Could you check a few things on this model? Use its own coordinates, in mm. Face numbers are marked on the shaded views. A direction names the side the tool comes from. Round coordinates to 2 decimals unless told otherwise and drop trailing zeros. Loops run counter-clockwise (first coordinate to the right, second up) from the corner with the lowest first, then second, coordinate; pieces in that order, holes last. Notation, with made-up numbers: M -7.5,67.25 L -1.5,67.25 A8 cw -1.5,78.25 Z; hole C 20,25 d8. An arc over 180 degrees is marked long. Answer in a Markdown table with one row per item.
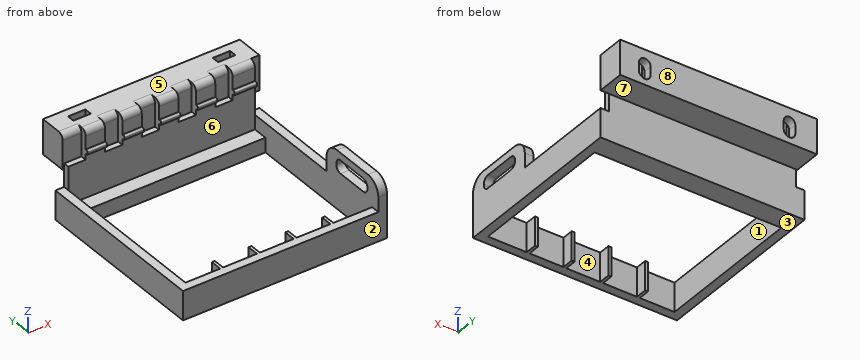
```python
from build123d import *

# Parameters (mm, degrees)
F0_W      = 70.5
F0_H      = 61.57
F0_W_2    = 1
F0_H_2    = 4
F1_DEPTH  = 10
F0_W_3    = 64.5
F0_H_3    = 5.07
F2_DEPTH  = 5
F3_W      = 64.5
F3_H      = 2
F4_DEPTH  = 18
F5_W      = 1
F5_H      = 1.5
F6_DEPTH  = 64.5
F7_R      = 0.5
F8_W      = 6
F8_H      = 9.142870052
F9_DEPTH  = 10
F10_W     = 9.5
F10_H     = 12
F11_DEPTH = 68
F13_DEPTH = 4
F14_W     = 6
F14_H     = 2.6
F15_DEPTH = 11
F17_DEPTH = 10
F18_W     = 15
F18_H     = 4.5
F19_DEPTH = 25
F20_R     = 5
F21_R     = 1.99999


# Not quite as in the source:
# - a fillet or chamfer is up to 0.001 mm smaller than in the source, because OpenCascade refuses the exact size


with BuildPart() as f1:
    # F0 (on Top) → F1 (new body)
    with BuildSketch(Plane.XY):
        with Locations((20.3630310733, 4.7424566842)):
            Rectangle(F0_W, F0_H)
        Polygon((-11.8869689267, 28.4574566842), (-11.8869689267, 33.5274566842), (52.6130310733, 33.5274566842), (52.6130310733, 28.4574566842), (52.6130310733, -23.0425433158), (39.2130310733, -23.0425433158), (38.2130310733, -23.0425433158), (26.5130310733, -23.0425433158), (25.5130310733, -23.0425433158), (13.8130310733, -23.0425433158), (12.8130310733, -23.0425433158), (1.1130310733, -23.0425433158), (0.1130310733, -23.0425433158), (-11.8869689267, -23.0425433158), align=None, mode=Mode.SUBTRACT)
        with Locations((0.6130310733, -21.0425433158)):
            Rectangle(F0_W_2, F0_H_2)
        with Locations((13.3130310733, -21.0425433158)):
            Rectangle(F0_W_2, F0_H_2)
        with Locations((26.0130310733, -21.0425433158)):
            Rectangle(F0_W_2, F0_H_2)
        with Locations((38.7130310733, -21.0425433158)):
            Rectangle(F0_W_2, F0_H_2)
    extrude(amount=F1_DEPTH)

    # F0 (on Top) → F2 (join)
    with BuildSketch(Plane.XY):
        with Locations((20.3630310733, 30.9924566842)):
            Rectangle(F0_W_3, F0_H_3)
    extrude(amount=F2_DEPTH)

    # F3 (on face) → F4 (join)
    with BuildSketch(Plane.XY.offset(10)):
        with Locations((20.3630310733, 34.5274566842)):
            Rectangle(F3_W, F3_H)
    extrude(amount=F4_DEPTH)

    # F5 (on face) → F6 (join)
    with BuildSketch(Plane.YZ.offset(52.6130310733)):
        with Locations((33.0274566842, 20.75)):
            Rectangle(F5_W, F5_H)
    extrude(amount=-F6_DEPTH)

    # F7
    f7_edges = [f1.edges().sort_by_distance(p)[0] for p in [
        (20.363031, 32.527457, 21.5),
        (20.363031, 32.527457, 20),
    ]]
    fillet(f7_edges, radius=F7_R)

    # F8 (on face) → F9 (cut)
    with BuildSketch(Plane.XY.offset(28)):
        with Locations((-8.8869689267, 30.9560216582)):
            Rectangle(F8_W, F8_H)
        with Locations((3.8130310733, 30.9560216582)):
            Rectangle(F8_W, F8_H)
        with Locations((16.5130310733, 30.9560216582)):
            Rectangle(F8_W, F8_H)
        with Locations((29.2130310733, 30.9560216582)):
            Rectangle(F8_W, F8_H)
        with Locations((41.9130310733, 30.9560216582)):
            Rectangle(F8_W, F8_H)
    extrude(amount=-F9_DEPTH, mode=Mode.SUBTRACT)

    # F10 (on face) → F11 (join)
    with BuildSketch(Plane.YZ.offset(55.6130310733)):
        with Locations((40.2774566842, 22)):
            Rectangle(F10_W, F10_H)
    extrude(amount=-F11_DEPTH)

    # F12 (on face) → F13 (cut)
    with BuildSketch(Plane(origin=(0, 45.0274566842, 0), x_dir=(-1, 0, 0), z_dir=(0, 1, 0))):
        with BuildLine():
            ThreePointArc((-48.4359067289, 21.5), (-48.9359067289, 20.8228756555), (-49.1130310733, 20))
            ThreePointArc((-49.1130310733, 20), (-47.1130310733, 18), (-45.1130310733, 20))
            ThreePointArc((-45.1130310733, 20), (-45.2901554178, 20.8228756555), (-45.7901554178, 21.5))
            ThreePointArc((-45.7901554178, 21.5), (-47.1130310733, 21), (-48.4359067289, 21.5))
        make_face()
        with BuildLine():
            Line((-49.1130310733, 23), (-49.1130310733, 20))
            ThreePointArc((-49.1130310733, 20), (-48.9359067289, 20.8228756555), (-48.4359067289, 21.5))
            ThreePointArc((-48.4359067289, 21.5), (-48.9359067289, 22.1771243445), (-49.1130310733, 23))
        make_face()
        with BuildLine():
            ThreePointArc((-45.7901554178, 21.5), (-45.2901554178, 20.8228756555), (-45.1130310733, 20))
            Line((-45.1130310733, 20), (-45.1130310733, 23))
            ThreePointArc((-45.1130310733, 23), (-45.2901554178, 22.1771243445), (-45.7901554178, 21.5))
        make_face()
        with BuildLine():
            ThreePointArc((-49.1130310733, 23), (-48.9359067289, 22.1771243445), (-48.4359067289, 21.5))
            ThreePointArc((-48.4359067289, 21.5), (-47.1130310733, 22), (-45.7901554178, 21.5))
            ThreePointArc((-45.7901554178, 21.5), (-45.2901554178, 22.1771243445), (-45.1130310733, 23))
            ThreePointArc((-45.1130310733, 23), (-47.1130310733, 25), (-49.1130310733, 23))
        make_face()
        with BuildLine():
            ThreePointArc((1.5640932711, 21.5), (1.0640932711, 20.8228756555), (0.8869689267, 20))
            ThreePointArc((0.8869689267, 20), (2.8869689267, 18), (4.8869689267, 20))
            ThreePointArc((4.8869689267, 20), (4.7098445822, 20.8228756555), (4.2098445822, 21.5))
            ThreePointArc((4.2098445822, 21.5), (2.8869689267, 21), (1.5640932711, 21.5))
        make_face()
        with BuildLine():
            Line((0.8869689267, 23), (0.8869689267, 20))
            ThreePointArc((0.8869689267, 20), (1.0640932711, 20.8228756555), (1.5640932711, 21.5))
            ThreePointArc((1.5640932711, 21.5), (1.0640932711, 22.1771243445), (0.8869689267, 23))
        make_face()
        with BuildLine():
            ThreePointArc((4.2098445822, 21.5), (4.7098445822, 20.8228756555), (4.8869689267, 20))
            Line((4.8869689267, 20), (4.8869689267, 23))
            ThreePointArc((4.8869689267, 23), (4.7098445822, 22.1771243445), (4.2098445822, 21.5))
        make_face()
        with BuildLine():
            ThreePointArc((0.8869689267, 23), (1.0640932711, 22.1771243445), (1.5640932711, 21.5))
            ThreePointArc((1.5640932711, 21.5), (2.8869689267, 22), (4.2098445822, 21.5))
            ThreePointArc((4.2098445822, 21.5), (4.7098445822, 22.1771243445), (4.8869689267, 23))
            ThreePointArc((4.8869689267, 23), (2.8869689267, 25), (0.8869689267, 23))
        make_face()
        with BuildLine():
            ThreePointArc((-45.7901554178, 21.5), (-47.1130310733, 22), (-48.4359067289, 21.5))
            ThreePointArc((-48.4359067289, 21.5), (-47.1130310733, 21), (-45.7901554178, 21.5))
        make_face()
        with BuildLine():
            ThreePointArc((4.2098445822, 21.5), (2.8869689267, 22), (1.5640932711, 21.5))
            ThreePointArc((1.5640932711, 21.5), (2.8869689267, 21), (4.2098445822, 21.5))
        make_face()
    extrude(amount=-F13_DEPTH, mode=Mode.SUBTRACT)

    # F14 (on face) → F15 (cut)
    with BuildSketch(Plane.XY.offset(28)):
        with Locations((-2.8869689267, 40.7274566842)):
            Rectangle(F14_W, F14_H)
        with Locations((47.1130310733, 40.7274566842)):
            Rectangle(F14_W, F14_H)
    extrude(amount=-F15_DEPTH, mode=Mode.SUBTRACT)

    # F16 (on face) → F17 (join)
    with BuildSketch(Plane.XY.offset(10)):
        Polygon((52.6130310733, -26.0425433158), (55.6130310733, -26.0425433158), (55.6130310733, -1.0425433158), (52.6130310733, -1.0425433158), (52.6130310733, -23.0425433158), align=None)
    extrude(amount=F17_DEPTH)

    # F18 (on face) → F19 (cut)
    with BuildSketch(Plane.YZ.offset(55.6130310733)):
        with Locations((-13.2769846171, 15.1880288571)):
            Rectangle(F18_W, F18_H)
    extrude(amount=-F19_DEPTH, mode=Mode.SUBTRACT)

    # F20
    f20_edges = [f1.edges().sort_by_distance(p)[0] for p in [
        (54.113031, -1.042543, 20),
        (54.113031, -26.042543, 20),
    ]]
    fillet(f20_edges, radius=F20_R)

    # F21 (radius 2 in the source; OpenCascade refuses exactly that, so slightly less here)
    f21_edges = [f1.edges().sort_by_distance(p)[0] for p in [
        (54.113031, -20.776985, 17.438029),
        (54.113031, -20.776985, 12.938029),
        (54.113031, -5.776985, 12.938029),
        (54.113031, -5.776985, 17.438029),
        (41.913031, 35.527457, 28),
        (48.763031, 33.527457, 28),
        (35.563031, 33.527457, 28),
        (29.213031, 35.527457, 28),
        (22.863031, 33.527457, 28),
        (16.513031, 35.527457, 28),
        (10.163031, 33.527457, 28),
        (3.813031, 35.527457, 28),
        (-2.536969, 33.527457, 28),
        (-9.136969, 35.527457, 28),
    ]]
    fillet(f21_edges, radius=F21_R)


solid = f1.part
```
1) I need wall thicknesses on line 1 (X direction, y = -6.5, z = 1.75); line 2 (Y direction, x = 17, z = 3.75); line 3 (Y direction, x = 49.5, z = 8.25). Which ranges of each line are inside material? Lowest first, please.
Computed:
| item | result |
|---|---|
| line 1 | x = -14.89 to -11.89, 52.61 to 55.61 |
| line 2 | y = -26.04 to -23.04, 28.46 to 35.53 |
| line 3 | y = -26.04 to -23.04, 33.53 to 35.53 |
2) Will these pins go through, and if not, where does the flat tip stop? P1, Ø2.5, axis at x = 54.5, z = 25, coming from the -Y side; P2, Ø0.5, axis at x = 26, z = 4.5, coming from the +Y side; P3, Ø2, axis at y = 40.5, z = 25, coming from the -X side; P4, Ø2, axis at y = 30, z = 21.5, coming from the +X side.
Computed:
| item | result |
|---|---|
| P1 | stops at y = 35.53 |
| P2 | stops at y = 35.53 |
| P3 | stops at x = -12.39 |
| P4 | passes through |
3) Which directions (+Z, -Z, +X, -X, +Y, -Y) give clear straight access to the entire face, cutting with the end or side of a thin tool? Please do the marked faces 4, 5, 6, 7 and 8.
Computed:
| item | result |
|---|---|
| face 4 | +Z, -Z |
| face 5 | +Z, +X, -X, +Y, -Y |
| face 6 | none |
| face 7 | -Z, +X, -X, +Y |
| face 8 | +Z, -Z, +X, -X, +Y |
4) I want a section at D-D, the plane x = 11.5. Please give me the cut outline in (y, z).
Computed:
| item | result |
|---|---|
| outline | M -26.04,0 L -23.04,0 L -23.04,10 L -26.04,10 Z; M 28.46,0 L 35.53,0 L 35.53,16 L 45.03,16 L 45.03,28 L 35.53,28 A2 ccw 33.53,26 L 33.53,21.5 L 33.03,21.5 A0.5 ccw 32.53,21 L 32.53,20.5 A0.5 ccw 33.03,20 L 33.53,20 L 33.53,5 L 28.46,5 Z |
5) I want a section at A-A, the plane x = -8.5. Please give me the cut outline in (y, z).
Computed:
| item | result |
|---|---|
| outline | M -26.04,0 L -23.04,0 L -23.04,10 L -26.04,10 Z; M 28.46,0 L 35.53,0 L 35.53,16 L 45.03,16 L 45.03,28 L 37.53,28 A2 ccw 35.53,26 L 35.53,18 L 33.53,18 L 33.53,5 L 28.46,5 Z |
6) I want a section at C-C, the plane y = -12. Please give me the cut outline in (x, z), plus the area to 3 significant figures.
Computed:
| item | result |
|---|---|
| outline | M -14.89,0 L -11.89,0 L -11.89,10 L -14.89,10 Z; M 52.61,0 L 55.61,0 L 55.61,12.94 L 52.61,12.94 Z; M 52.61,17.44 L 55.61,17.44 L 55.61,20 L 52.61,20 Z |
| area | 76.5 mm² |
7) If we mould it in two halves opening along Y, with no side actions, what happens to the marked faces 1, 2 and 3? For each: released by +Y, released by -Y, zero draft, split by the parting line, or undercut.
Computed:
| item | result |
|---|---|
| face 1 | undercut |
| face 2 | released by -Y |
| face 3 | zero draft |
8) I want a section at B-B, the plane y = 27.5. Please give me the cut outline in (x, z), plus the area to 3 significant figures.
Computed:
| item | result |
|---|---|
| outline | M -14.89,0 L -11.89,0 L -11.89,10 L -14.89,10 Z; M 52.61,0 L 55.61,0 L 55.61,10 L 52.61,10 Z |
| area | 60.0 mm² |
